```python
from build123d import *

# Parameters (mm, degrees)
F0_W     = 93.4118106961
F0_H     = 75.4010342062
F1_DEPTH = 25.4
F2_SIZE  = 5.08
F3_R     = 5.08
F4_T     = -2.54


# Not quite as in the source:
# - a shell that OpenCascade refuses in one call is made with other operations: the cavity is built on its own and cut out


with BuildPart() as f1:
    # F0 (on Front) → F1 (new body)
    with BuildSketch(Plane.XZ):
        with Locations((0.4579015076, -3.3579412848)):
            Rectangle(F0_W, F0_H)
    extrude(amount=F1_DEPTH)

    # F2
    f2_edges = [f1.edges().sort_by_distance(p)[0] for p in [
        (0.457902, -25.4, 34.342576),
        (-46.248004, -25.4, -3.357941),
        (0.457902, -25.4, -41.058458),
        (47.163807, -25.4, -3.357941),
    ]]
    chamfer(f2_edges, length=F2_SIZE)

    # F3
    f3_edges = [f1.edges().sort_by_distance(p)[0] for p in [
        (0.457902, -25.4, 29.262576),
        (42.083807, -25.4, -3.357941),
        (-41.168004, -25.4, -3.357941),
        (0.457902, -25.4, -35.978458),
    ]]
    fillet(f3_edges, radius=F3_R)

    # F4: a shell. OpenCascade refuses it in one call, so the cavity is built on its own and cut out:
    # the body offset inwards by the wall thickness, plus a prism from it out through each open face.
    f4_core = offset(f1.part, amount=F4_T, mode=Mode.PRIVATE)
    f4_exits = [f4_core.faces().sort_by_distance(p)[0] for p in [
        (0.457902, -22.86, -3.357941),
    ]]
    add(f4_core, mode=Mode.SUBTRACT)
    extrude(f4_exits, amount=-F4_T, mode=Mode.SUBTRACT)


solid = f1.part
```
Check sheet for the modelled part. Datum: model origin and axes. Units: mm. A direction names the side the tool comes from. Coordinates: 2 decimals unless noted, no trailing zeros. Write each loop counter-clockwise with the first axis right and the second up, starting at its lowest first coordinate (ties: lowest second). Pieces come first, ordered by that corner, then holes. Notation, with made-up numbers: (81, 47) -> (111, 47) arc R17 cw to (111, 76) -> close; hole circle Ø3 at (76, 41). An arc over 180 degrees is marked (long way). Use a Markdown table: item, result.
1. Tool access check on faces 1 (the flat face through (39.98, -24, -4)), 2 (the flat face through (0, 0, -3)), 3 (the flat face through (-43.708, -11, -4)). Record the directions out of +Z, -Z, +X, -X, +Y, -Y that give a thin tool (end or side, any length) a straight path to the whole face; none if there is none.
Reported:
| item | result |
|---|---|
| face 1 | -Y |
| face 2 | +Z, -Z, +X, -X, +Y |
| face 3 | none |
2. Release check for a two-part mould opening along X. For faces 4 (the cylindrical face through (41.898, -25.024, -2.88)), 5 (the flat face through (0, -11, -38.518)), 6 (the cylindrical face through (1.061, -25.024, 29.077)), 7 (the flat face through (-44.43, -22.14, -3.89)) record: pulls with the +X half, pulls with the -X half, needs draft (parallel to the pull), parting line crosses it, or undercut.
Reported:
| item | result |
|---|---|
| face 4 | pulls with the +X half |
| face 5 | undercut |
| face 6 | needs draft |
| face 7 | pulls with the -X half |
3. Sectioned sample at C-C (z = 0.5). Enter the section's corners in (x, y).
Reported:
| item | result |
|---|---|
| outline | (-46.25, -20.32) -> (-42.66, -23.91) arc R5.08 ccw to (-39.06, -25.4) -> (-39.06, -22.86) arc R2.54 cw to (-40.86, -22.12) -> (-43.71, -19.27) -> (-43.71, -2.54) -> (44.62, -2.54) -> (44.62, -19.27) -> (41.78, -22.12) arc R2.54 cw to (39.98, -22.86) -> (39.98, -25.4) arc R5.08 ccw to (43.57, -23.91) -> (47.16, -20.32) -> (47.16, 0) -> (-46.25, 0) -> close |
4. Sectioned sample at B-B (x = -1). Enter the section's corners in (y, z), plus the area to 3 significant figures.
Reported:
| item | result |
|---|---|
| outline | (-25.4, -33.87) arc R5.08 ccw to (-23.91, -37.47) -> (-20.32, -41.06) -> (0, -41.06) -> (0, 34.34) -> (-20.32, 34.34) -> (-23.91, 30.75) arc R5.08 ccw to (-25.4, 27.16) -> (-22.86, 27.16) arc R2.54 cw to (-22.12, 28.95) -> (-19.27, 31.8) -> (-2.54, 31.8) -> (-2.54, -38.52) -> (-19.27, -38.52) -> (-22.12, -35.67) arc R2.54 cw to (-22.86, -33.87) -> close |
| area | 318 mm2 |
5. Go/stop test with flat-tipped pins: pin 1 Ø4 at (x, z) = (3.5, -32.5) entering from +Y; pin 2 Ø1.3 at (x, y) = (-2.5, -24) entering from +Z; pin 3 Ø0.8 at (y, z) = (-24.5, 10) entering from -X; pin 4 Ø3 at (x, y) = (2.5, -24) entering from -Z. Record where each tip stops, or that it passes through.
Reported:
| item | result |
|---|---|
| pin 1 | stops at y = 0 |
| pin 2 | stops at z = 31.31 |
| pin 3 | stops at x = -42.46 |
| pin 4 | stops at z = -38.88 |
6. Sectioned sample at A-A (y = -14). Enter the section's corners in (x, z).
Reported:
| item | result |
|---|---|
| outline | (-46.25, -41.06) -> (47.16, -41.06) -> (47.16, 34.34) -> (-46.25, 34.34) -> close; hole (-43.71, -38.52) -> (44.62, -38.52) -> (44.62, 31.8) -> (-43.71, 31.8) -> close |
7. Scan lines: line 1 along Z through (x, y) = (1.5, -16.5); line 2 along X through (y, z) = (-6.75, -1); line 3 along Z through (x, y) = (-27, -22). Record each from-to range of solid material in increasing order.
Reported:
| item | result |
|---|---|
| line 1 | z = -41.06 to -38.52, 31.8 to 34.34 |
| line 2 | x = -46.25 to -43.71, 44.62 to 47.16 |
| line 3 | z = -39.38 to -35.79, 29.07 to 32.66 |
